Geometry check sheet. Reference: drawing and pictorial views, mm from the part's lowest x, y, z. A direction names the side the tool comes from. Give positions to 0.01 mm unless a question says otherwise; leave off trailing zeros. Order: outer loops, then holes, each group sorted by start corner. A loop starts at its lowest first (then second) coordinate and runs counter-clockwise, first axis right, second up. Notation, with made-up numbers: (-4, 14) -> (26, 14) arc R31 ccw to (26, 47) -> close; hole circle Ø2 at (68, 80). An arc over 180 degrees is marked (long way). Write each question's results on one line, items separated by ' | '.
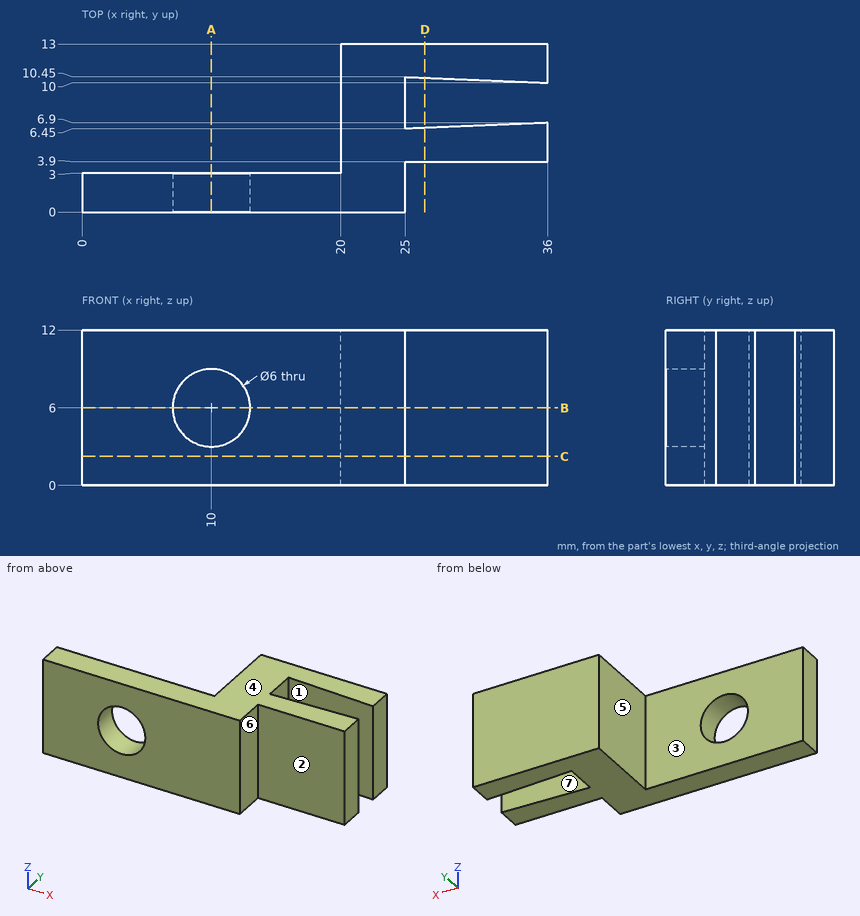
1. Mould release check, pull along X, two halves, no side actions. Record for the marked faces 5, 6 and 7: +X half, -X half, draft (parallel to the pull), parting line (faces both ways), or undercut.
Verdict:
face 5: -X half | face 6: +X half | face 7: undercut
2. Section check C-C on z = 2.25. Record the cut outline in (x, y).
Verdict:
outline: (0, 0) -> (25, 0) -> (25, 3.9) -> (36, 3.9) -> (36, 6.9) -> (25, 6.45) -> (25, 10.45) -> (36, 10) -> (36, 13) -> (20, 13) -> (20, 3) -> (0, 3) -> close
3. Section check D-D on x = 26.5. Record the cut outline in (y, z).
Verdict:
outline: (3.9, 0) -> (6.51, 0) -> (6.51, 12) -> (3.9, 12) -> close; (10.39, 0) -> (13, 0) -> (13, 12) -> (10.39, 12) -> close
4. Access from +Z, -Z, +X, -X, +Y, -Y to the whole of each face (thin tool, end or side, straight path). Record for the marked faces 1, 2, 3 and 4.
Verdict:
face 1: +Z, -Z | face 2: +Z, -Z, +X, -Y | face 3: +Z, -Z, -X, +Y | face 4: +Z, +X, -X, +Y, -Y
5. Section check A-A on x = 10. Record the cut outline in (y, z), then the cut area to 3 significant figures.
Verdict:
outline: (0, 0) -> (3, 0) -> (3, 3) -> (0, 3) -> close; (0, 9) -> (3, 9) -> (3, 12) -> (0, 12) -> close | area: 18.0 mm^2
6. Gauge pin test, flat ends, axial feed: pin 1 Ø4 at (x, y) = (16.5, 11.5) entering from +Z; pin 2 Ø6 at (x, z) = (9, 8) entering from +Y; pin 3 Ø1.2 at (y, z) = (9, 7) entering from +X. Record the tip position at first contact, or that the pin passes through.
Verdict:
pin 1: passes through | pin 2: stops at y = 3 | pin 3: stops at x = 25
7. Material ranges on probe 1 along Z at (x, y) = (10, 1.2); probe 2 along X at (y, z) = (3.5, 0.75); probe 3 along X at (y, z) = (12, 3), recorded low to high. Write a range as from..to.
Verdict:
probe 1: z = 0..3, 9..12 | probe 2: x = 20..25 | probe 3: x = 20..36
8. Section check B-B on z = 6. Record the cut outline in (x, y).
Verdict:
outline: (0, 0) -> (7, 0) -> (7, 3) -> (0, 3) -> close; (13, 0) -> (25, 0) -> (25, 3.9) -> (36, 3.9) -> (36, 6.9) -> (25, 6.45) -> (25, 10.45) -> (36, 10) -> (36, 13) -> (20, 13) -> (20, 3) -> (13, 3) -> close
